For this review, take the finished solid that the model builds, in its own axes (mm). A direction names the side the tool comes from. Give positions to 0.01 mm unless a question says otherwise; leave off trailing zeros. Write each loop counter-clockwise with the first axis right and the second up, starting at its lowest first coordinate (ties: lowest second). Pieces come first, ordered by that corner, then holes. Notation, with made-up numbers: (44.25, 65.5) -> (60.25, 65.5) arc R29 cw to (60.25, 93.5) -> close; hole circle Ø11 at (48.25, 60.5). An arc over 180 degrees is marked (long way). Return JSON: item names as keys, results as strings.
from build123d import *

# Parameters (mm, degrees)
BOSS_EXTRUDE1_DEPTH = 32
SKETCH2_R           = 6.5
CUT_EXTRUDE1_DEPTH  = 32
SKETCH3_R           = 6.5
CUT_EXTRUDE2_DEPTH  = 76
CUT_EXTRUDE5_START  = -63
CUT_EXTRUDE5_DEPTH  = 63


# Read off the part's stored shape, not the designer's step: Cut-Extrude5
with BuildPart() as part:
    # Sketch1 → Boss-Extrude1 (new body)
    with BuildSketch(Plane.XY):
        Polygon((-64.877213136, -12.117917581), (-64.877213136, -25.117917581), (-26.877213136, -25.117917581), (-26.877213136, -8.117917581), (8.122786864, -8.117917581), (8.122786864, -25.117917581), (48.122786864, -25.117917581), (48.122786864, -12.117917581), (23.122786864, -12.117917581), (23.122786864, 38.882082419), (4.122786864, 38.882082419), (4.122786864, 4.882082419), (-20.877213136, 4.882082419), (-20.877213136, 38.882082419), (-39.877213136, 38.882082419), (-39.877213136, -12.117917581), align=None)
    extrude(amount=BOSS_EXTRUDE1_DEPTH)

    # Sketch2 → Cut-Extrude1 (cut)
    with BuildSketch(Plane(origin=(0, -12.117917581, 0), x_dir=(1, 0, 0), z_dir=(0, 1, 0))):
        with Locations(Location((35.122786864, -13, 0), (0, 0, 180))):
            Circle(SKETCH2_R)
        with Locations(Location((-51.877213136, -13, 0), (0, 0, 270))):
            Circle(SKETCH2_R)
    extrude(amount=-CUT_EXTRUDE1_DEPTH, mode=Mode.SUBTRACT)

    # Sketch3 → Cut-Extrude2 (cut)
    with BuildSketch(Plane.ZY.offset(39.877213136)):
        with Locations(Location((16, 20.882082419, 0), (0, 0, 270))):
            Circle(SKETCH3_R)
    extrude(amount=-CUT_EXTRUDE2_DEPTH, mode=Mode.SUBTRACT)

    # Cut-Extrude5 outline → Cut-Extrude5 (cut)
    with BuildSketch(Plane(origin=(23.122786864, 0, 0), x_dir=(0, 0, -1), z_dir=(1, 0, 0)).offset(CUT_EXTRUDE5_START)):
        with BuildLine():
            ThreePointArc((-32, 35.010847251), (-24.230833216, 37.900509551), (-16, 38.882082419))
            Line((-16, 38.882082419), (-32, 38.882082419))
            Line((-32, 38.882082419), (-32, 35.010847251))
        make_face()
        with BuildLine():
            ThreePointArc((-16, 38.882082419), (-7.769166784, 37.900509551), (0, 35.010847251))
            Line((0, 35.010847251), (0, 38.882082419))
            Line((0, 38.882082419), (-16, 38.882082419))
        make_face()
    extrude(amount=CUT_EXTRUDE5_DEPTH, mode=Mode.SUBTRACT)


solid = part.part
1. Add section A-A, the plane y = -10. State the section outline as (x, z) points.
Results found:
{"outline": "(-39.88, 0) -> (-26.88, 0) -> (-26.88, 32) -> (-39.88, 32) -> close; (8.12, 0) -> (23.12, 0) -> (23.12, 32) -> (8.12, 32) -> close"}
2. To check wall thickness, follow probe 1 along X at (y, z) = (-16.5, 1.5); probe 2 along X at (y, z) = (12, 27.5); probe 3 along X at (y, z) = (4.5, 20). State the ranges of each line that lie inside material, in increasing order.
Results found:
{"probe 1": "x = -64.88 to -26.88, 8.12 to 48.12", "probe 2": "x = -39.88 to -20.88, 4.12 to 23.12", "probe 3": "x = -39.88 to 23.12"}
3. For pin 1 (3 mm diameter, centred on y = 22.5, z = 27, fed in from -X); pin 2 (15 mm diameter, centred on x = -51.88, z = 13, fed in from -Y); pin 3 (4 mm diameter, centred on x = -13.5, z = 16, fed in from +Y); pin 4 (16 mm diameter, centred on y = 23, z = 17.5, fed in from +X), all flat-tipped, find the tip position at first contact; note any pin that passes through.
Results found:
{"pin 1": "stops at x = -39.88", "pin 2": "stops at y = -25.12", "pin 3": "stops at y = 4.88", "pin 4": "stops at x = 23.12"}
4. Add section B-B, the plane x = 19. State the section outline as (y, z) points.
Results found:
{"outline": "(-25.12, 0) -> (35.01, 0) arc R35 ccw to (35.01, 32) -> (-25.12, 32) -> close; hole circle Ø13 at (20.88, 16)"}
5. For faces 4 (the flat face through (-8, 4.882, 16)), 5 (the flat face through (-26.877, -17, 16)), 6 (the flat face through (23.123, 13, 16)), list the 3-axis set-ups (+Z, -Z, +X, -X, +Y, -Y) from which the entire face can be reached by the end or side of a thin tool; tool diameter is ignored.
Results found:
{"face 4": "+Z, -Z, +Y", "face 5": "+Z, -Z, -Y", "face 6": "+Z, -Z, +X, +Y"}
6. The part is to be moulded in two halves that separate along Y. For faces 1 (the cylindrical face through (13.49, 21.728, 22.445)), 2 (the flat face through (-55, -12.118, 19)), 3 (the flat face through (-9, -1, 32)), say which applies: +Y half, -Y half, draft (parallel to the pull), parting line (faces both ways), or undercut.
Results found:
{"face 1": "undercut", "face 2": "+Y half", "face 3": "draft"}
7. Add section D-D, the plane z = 3. State the section outline as (x, y) points, plus the area to 3 significant figures.
Results found:
{"outline": "(-64.88, -25.12) -> (-26.88, -25.12) -> (-26.88, -8.12) -> (8.12, -8.12) -> (8.12, -25.12) -> (48.12, -25.12) -> (48.12, -12.12) -> (23.12, -12.12) -> (23.12, 36.38) -> (4.12, 36.38) -> (4.12, 4.88) -> (-20.88, 4.88) -> (-20.88, 36.38) -> (-39.88, 36.38) -> (-39.88, -12.12) -> (-64.88, -12.12) -> close", "area": "3,140 mm²"}
8. Add section C-C, the plane z = 13. Count the separate pieces of the cut face and the enclosed holes in it, plus the area to 3 significant figures.
Results found:
{"separate pieces": "5", "enclosed holes": "0", "area": "2,460 mm²"}
